Model file for the job. Use its own axes, mm. A direction names the side the tool comes from. Give positions to 0.01 mm unless a question says otherwise; leave off trailing zeros. Loops run counter-clockwise (first coordinate to the right, second up) from the corner with the lowest first, then second, coordinate; pieces in that order, holes last. Notation, with made-up numbers: M 81.25,70.25 L 95.25,70.25 A23 ccw 95.25,95.25 Z; hole C 34.5,-14 d7. An arc over 180 degrees is marked long. Answer in a Markdown table with one row per item.
```python
from build123d import *

# Parameters (mm, degrees)
F1_DEPTH = 38.1
F3_DEPTH = 152.4
F4_W     = 53.3399991691
F4_H     = 7.4427900836
F5_DEPTH = 152.4


with BuildPart() as f1:
    # F0 (on Top) → F1 (new body)
    with BuildSketch(Plane.XY):
        with BuildLine():
            ThreePointArc((-47.6478643498, -0.3401276624), (-53.0503273428, 10.0446370996), (-48.3781397343, 20.7777917385))
            ThreePointArc((-48.3781397343, 20.7777917385), (-68.74194328, -1.5809564376), (-45.8972081542, -21.3980246335))
            Line((-45.8972081542, -21.3980246335), (-45.8972081542, -62.0232559741))
            Line((-45.8972081542, -62.0232559741), (53.6501146853, -62.0232559741))
            Line((53.6501146853, -62.0232559741), (51.7894178629, -20.4676743597))
            ThreePointArc((51.7894178629, -20.4676743597), (65.7973197018, 1.4426008353), (48.0680204928, 20.4676743597))
            ThreePointArc((48.0680204928, 20.4676743597), (55.2873850052, 8.5442586778), (44.6631883311, -0.4786848838))
            Line((44.6631883311, -0.4786848838), (-47.6478643498, -0.3401276624))
        make_face()
    extrude(amount=F1_DEPTH)

    # F2 (on face) → F3 (cut)
    with BuildSketch(Plane(origin=(50.7711641994, 2.2733346575, 0), x_dir=(-0.0447312803, 0.9989990553, 0), z_dir=(0.9989990553, 0.0447312803, 0))):
        with BuildLine():
            Line((-64.3610124434, 38.1), (-64.3610124434, 0))
            ThreePointArc((-64.3610124434, 0), (-45.3110124434, 19.05), (-64.3610124434, 38.1))
        make_face()
    extrude(amount=-F3_DEPTH, mode=Mode.SUBTRACT)

    # F4 (on face) → F5 (cut)
    with BuildSketch(Plane.XY.offset(38.1)):
        with Locations((0, -6.8225585856)):
            Rectangle(F4_W, F4_H)
    extrude(amount=-F5_DEPTH, mode=Mode.SUBTRACT)


solid = f1.part
```
Q1. Drop flat-ended pins along their axis: pin 1 (1.5 mm diameter, centred on x = -23, z = 11.5, fed in from +Y); pin 2 (11.5 mm diameter, centred on y = -43, z = 16, fed in from -X); pin 3 (11.5 mm diameter, centred on x = -9, z = 25, fed in from -Y). Give the stop position or say it passes through.
Reported:
| item | result |
|---|---|
| pin 1 | y = -0.38 |
| pin 2 | x = -45.9 |
| pin 3 | y = -49.79 |
Q2. Saw through at B-B (y = -9). Give the cut face in (x, z), and give its area (3 significant figures).
Reported:
| item | result |
|---|---|
| outline | M -66.92,0 L -26.67,0 L -26.67,38.1 L -66.92,38.1 Z; M 26.67,0 L 64.1,0 L 64.1,38.1 L 26.67,38.1 Z |
| area | 2,960 mm² |
Q3. Saw through at D-D (z = 34). Give the cut face in (x, y).
Reported:
| item | result |
|---|---|
| outline | M -48.38,20.78 A21.13 ccw long -45.9,-21.4 L -45.9,-54.66 L 53.12,-50.23 L 51.79,-20.47 A21.22 ccw 48.07,20.47 A10.75 cw 44.66,-0.48 L -47.65,-0.34 A13.59 cw Z; hole M -26.67,-10.54 L 26.67,-10.54 L 26.67,-3.1 L -26.67,-3.1 Z |
Q4. Mould opens along X. For faces 1 (the face through (-2, -29, 38.1)), 2 (the face through (65.83, 1.05, 18.78)), 3 (the face through (26.67, -7, 19)) say: released by +X, released by -X, zero draft, split by the parting line, or undercut.
Reported:
| item | result |
|---|---|
| face 1 | zero draft |
| face 2 | released by +X |
| face 3 | undercut |
Q5. Saw through at C-C (z = 14). Give the cut face in (x, y).
Reported:
| item | result |
|---|---|
| outline | M -48.38,20.78 A21.13 ccw long -45.9,-21.4 L -45.9,-48.09 L 52.83,-43.67 L 51.79,-20.47 A21.22 ccw 48.07,20.47 A10.75 cw 44.66,-0.48 L -47.65,-0.34 A13.59 cw Z; hole M -26.67,-10.54 L 26.67,-10.54 L 26.67,-3.1 L -26.67,-3.1 Z |
Q6. 3-axis set-ups, long thin cutter, end or side, ignore diameter. For faces 4 (the face through (52.32, -32.3, 18.78)), 5 (the face through (-53.043, 9.875, 18.783)), 6 (the face through (-2, -29, 0)): which of +Z, -Z, +X, -X, +Y, -Y reach the whole face in a straight line?
Reported:
| item | result |
|---|---|
| face 4 | +Z, -Z, +X |
| face 5 | +Z, -Z |
| face 6 | -Z, +X, -X, +Y, -Y |
Q7. Saw through at A-A (x = -51.5). Give the cut face in (y, z).
Reported:
| item | result |
|---|---|
| outline | M -21.12,0 L 4.19,0 L 4.19,38.1 L -21.12,38.1 Z; M 16.83,0 L 20.44,0 L 20.44,38.1 L 16.83,38.1 Z |
Q8. Probe probe 1 along Y at (x, z) = (51.5, 15); probe 2 along Y at (x, z) = (22, 29.5); probe 3 along X at (y, z) = (-3.5, 3.5). List the from-to ranges inside material, lowest first.
Reported:
| item | result |
|---|---|
| probe 1 | -43.49 to 1.96, 18.57 to 19.61 |
| probe 2 | -47.5 to -10.54, -3.1 to -0.44 |
| probe 3 | -68.54 to -26.67, 26.67 to 65.67 |
